The model under review builds one solid part; all positions refer to its coordinate system, in mm. A direction names the side the tool comes from. Coordinates: 2 decimals unless noted, no trailing zeros. Loops run counter-clockwise (first coordinate to the right, second up) from the corner with the lowest first, then second, coordinate; pieces in that order, holes last. Notation, with made-up numbers: M -27.75,-37 L -3.75,-37 A13 cw -3.75,-21 Z; hole C 47,6.5 d4. An arc over 180 degrees is marked long. Use one line per item in the form item = value.
```python
from build123d import *

# Parameters (mm, degrees)
SKETCH1_W                                            = 59.1
SKETCH1_H                                            = 59.1
BOSS_EXTRUDE1_DEPTH                                  = 59.1
CUT_EXTRUDE1_START                                   = -2.25
SKETCH2_W                                            = 116.357411776
SKETCH2_H                                            = 94.431830133
CUT_EXTRUDE1_DEPTH                                   = 71.232302632
FILLET1_R                                            = 7.5
SHELL1_T                                             = -2.5
CUT_EXTRUDE7_DEPTH                                   = 35
CUT_EXTRUDE8_DEPTH                                   = 35
SKETCH16_W                                           = 0.690169944
SKETCH16_H                                           = 5
CUT_EXTRUDE9_DEPTH                                   = 88.003290168
BOSS_EXTRUDE2_START                                  = 3
SKETCH18_R                                           = 5
BOSS_EXTRUDE2_DEPTH                                  = 3
SKETCH17_R                                           = 1.5
CUT_EXTRUDE10_DEPTH                                  = 10
CUT_EXTRUDE11_REACH                                  = 90.65
CSK_SLOT_FOR_M2_COUNTERSUNK_FLAT_HEAD_SC_D           = 2.4
CSK_SLOT_FOR_M2_COUNTERSUNK_FLAT_HEAD_SC_CSINK_D     = 4.4
CSK_SLOT_FOR_M2_COUNTERSUNK_FLAT_HEAD_SC_CSINK_ANGLE = 90
CSK_SLOT_FOR_M2_COUNTERSUNK_FLAT_HEA_2_D             = 2.4
CSK_SLOT_FOR_M2_COUNTERSUNK_FLAT_HEA_2_CSINK_D       = 4.4
CSK_SLOT_FOR_M2_COUNTERSUNK_FLAT_HEA_2_CSINK_ANGLE   = 90
CSK_SLOT_FOR_M2_COUNTERSUNK_FLAT_HEA_3_D             = 2.4
CSK_SLOT_FOR_M2_COUNTERSUNK_FLAT_HEA_3_CSINK_D       = 4.4
CSK_SLOT_FOR_M2_COUNTERSUNK_FLAT_HEA_3_CSINK_ANGLE   = 90
BOSS_EXTRUDE3_DEPTH                                  = 35
SKETCH28_W                                           = 7.5
SKETCH28_H                                           = 5.1
CUT_EXTRUDE12_DEPTH                                  = 62.984090748


with BuildPart() as part:
    # Sketch1 → Boss-Extrude1 (new body)
    with BuildSketch(Plane.XY):
        Rectangle(SKETCH1_W, SKETCH1_H)
    extrude(amount=BOSS_EXTRUDE1_DEPTH)

    # Sketch2 → Cut-Extrude1 (cut, through all)
    with BuildSketch(Plane(origin=(-13.400446417, -13.400446417, 19.55), x_dir=(0.9659258262890684, -0.2588190451025203, 0), z_dir=(0, 0, 1)).offset(CUT_EXTRUDE1_START)):
        with Locations((15.241895832, 15.980077556)):
            Rectangle(SKETCH2_W, SKETCH2_H)
    extrude(amount=-CUT_EXTRUDE1_DEPTH, mode=Mode.SUBTRACT)

    # Fillet1
    fillet1_edges = [part.edges().sort_by_distance(p)[0] for p in [
        (29.55, 0, 59.1),
        (0, 29.55, 59.1),
        (-29.55, 0, 59.1),
        (0, -29.55, 59.1),
        (-29.55, 29.55, 38.2),
        (29.55, 29.55, 38.2),
        (29.55, -29.55, 38.2),
        (-29.55, -29.55, 38.2),
    ]]
    fillet(fillet1_edges, radius=FILLET1_R)

    # Shell1
    shell1_openings = [part.faces().sort_by_distance(p)[0] for p in [
        (0, 0, 17.3),
    ]]
    offset(amount=SHELL1_T, openings=shell1_openings, kind=Kind.INTERSECTION)

    # Sketch14 → Cut-Extrude7 (cut)
    with BuildSketch(Plane.XY.offset(59.1)):
        Polygon((-29.55, -8.7), (-27.05, -8.7), (-27.05, -7.5), (-24.55, -7.5), (-24.55, -12.5), (-27.05, -12.5), (-27.05, -11.3), (-29.55, -11.3), align=None)
        Polygon((-29.55, 11.3), (-29.55, 8.7), (-27.05, 8.7), (-27.05, 7.5), (-24.55, 7.5), (-24.55, 12.5), (-27.05, 12.5), (-27.05, 11.3), align=None)
    extrude(amount=-CUT_EXTRUDE7_DEPTH, mode=Mode.SUBTRACT)

    # Sketch15 → Cut-Extrude8 (cut)
    with BuildSketch(Plane(origin=(-29.55, 0, -29.55), x_dir=(0, 0, -1), z_dir=(1, 0, 0))):
        Polygon((-88.65, -8.7), (-86.05, -8.7), (-86.05, -7.5), (-83.45, -7.5), (-83.45, -12.5), (-86.05, -12.5), (-86.05, -11.3), (-88.65, -11.3), align=None)
        Polygon((-88.65, 11.3), (-88.65, 8.7), (-86.05, 8.7), (-86.05, 7.5), (-83.45, 7.5), (-83.45, 12.5), (-86.05, 12.5), (-86.05, 11.3), align=None)
    extrude(amount=CUT_EXTRUDE8_DEPTH, mode=Mode.SUBTRACT)

    # Sketch16 → Cut-Extrude9 (cut, through all)
    with BuildSketch(Plane(origin=(-27.05, 0, 0), x_dir=(0, 0, -1), z_dir=(1, 0, 0))):
        with Locations((-56.845084972, -10)):
            Rectangle(SKETCH16_W, SKETCH16_H)
        with Locations((-56.845084972, 10)):
            Rectangle(SKETCH16_W, SKETCH16_H)
    extrude(amount=-CUT_EXTRUDE9_DEPTH, mode=Mode.SUBTRACT)

    # Sketch18 → Boss-Extrude2 (add)
    with BuildSketch(Plane(origin=(0, -27.05, 0), x_dir=(1, 0, 0), z_dir=(0, 1, 0)).offset(BOSS_EXTRUDE2_START)):
        with Locations((-22.05, -51.6)):
            Circle(SKETCH18_R)
    extrude(amount=-BOSS_EXTRUDE2_DEPTH)

    # Sketch17 → Cut-Extrude10 (cut)
    with BuildSketch(Plane.XZ.offset(29.55)):
        with Locations(Location((-22.05, 51.6, 0), (0, 0, 90))):
            Circle(SKETCH17_R)
    extrude(amount=-CUT_EXTRUDE10_DEPTH, mode=Mode.SUBTRACT)

    # Sketch20 → Cut-Extrude11 (cut, up to next)
    with BuildSketch(Plane.XZ.offset(29.55), mode=Mode.PRIVATE) as cut_extrude11_sk1:
        with BuildLine():
            Line((-22.647878988, 52.975696447), (-23.072143057, 53.399960516))
            Line((-23.072143057, 53.399960516), (-23.849960516, 52.622143057))
            Line((-23.849960516, 52.622143057), (-23.425696447, 52.197878988))
            ThreePointArc((-23.425696447, 52.197878988), (-23.110660172, 52.660660172), (-22.647878988, 52.975696447))
        make_face()
    cut_extrude11_tool1 = extrude(cut_extrude11_sk1.sketch, amount=-CUT_EXTRUDE11_REACH, mode=Mode.PRIVATE) & part.part
    # Sketch20 → Cut-Extrude11 (cut, up to next)
    with BuildSketch(Plane.XZ.offset(29.55), mode=Mode.PRIVATE) as cut_extrude11_sk2:
        with BuildLine():
            Line((-21.027856943, 49.800039484), (-21.452121012, 50.224303553))
            ThreePointArc((-21.452121012, 50.224303553), (-20.989339828, 50.539339828), (-20.674303553, 51.002121012))
            Line((-20.674303553, 51.002121012), (-20.250039484, 50.577856943))
            Line((-20.250039484, 50.577856943), (-21.027856943, 49.800039484))
        make_face()
    cut_extrude11_tool2 = extrude(cut_extrude11_sk2.sketch, amount=-CUT_EXTRUDE11_REACH, mode=Mode.PRIVATE) & part.part
    add(cut_extrude11_tool1.solids().sort_by_distance((-23.27308, -29.55, 52.82308))[0], mode=Mode.SUBTRACT)
    add(cut_extrude11_tool2.solids().sort_by_distance((-20.82692, -29.55, 50.37692))[0], mode=Mode.SUBTRACT)

    # CSK SLOT for M2 Countersunk Flat Head Sc (through all)
    with Locations(Plane.ZX.offset(29.55)):
        with Locations((29.55, 0)):
            CounterSinkHole(CSK_SLOT_FOR_M2_COUNTERSUNK_FLAT_HEAD_SC_D / 2, CSK_SLOT_FOR_M2_COUNTERSUNK_FLAT_HEAD_SC_CSINK_D / 2, counter_sink_angle=CSK_SLOT_FOR_M2_COUNTERSUNK_FLAT_HEAD_SC_CSINK_ANGLE)

    # CSK SLOT for M2 Countersunk Flat Hea 2 (through all)
    with Locations(Plane.XY.offset(59.1)):
        with Locations((0, 0)):
            CounterSinkHole(CSK_SLOT_FOR_M2_COUNTERSUNK_FLAT_HEA_2_D / 2, CSK_SLOT_FOR_M2_COUNTERSUNK_FLAT_HEA_2_CSINK_D / 2, counter_sink_angle=CSK_SLOT_FOR_M2_COUNTERSUNK_FLAT_HEA_2_CSINK_ANGLE)

    # CSK SLOT for M2 Countersunk Flat Hea 3 (through all)
    with Locations(Plane(origin=(0, -29.55, 0), x_dir=(-1, 0, 0), z_dir=(0, -1, 0))):
        with Locations((0, -29.55)):
            CounterSinkHole(CSK_SLOT_FOR_M2_COUNTERSUNK_FLAT_HEA_3_D / 2, CSK_SLOT_FOR_M2_COUNTERSUNK_FLAT_HEA_3_CSINK_D / 2, counter_sink_angle=CSK_SLOT_FOR_M2_COUNTERSUNK_FLAT_HEA_3_CSINK_ANGLE)

    # Sketch27 → Boss-Extrude3 (add)
    with BuildSketch(Plane(origin=(-29.55, 29.55, 0), x_dir=(0, 0, -1), z_dir=(1, 0, 0))):
        Polygon((-18.3, -59.1), (-18.3, -61.7), (-17.05, -61.7), (-17.05, -64.2), (-22.05, -64.2), (-22.05, -61.7), (-20.8, -61.7), (-20.8, -59.1), align=None)
        Polygon((-38.3, -59.1), (-40.8, -59.1), (-40.8, -61.7), (-42.05, -61.7), (-42.05, -64.2), (-37.05, -64.2), (-37.05, -61.7), (-38.3, -61.7), align=None)
    extrude(amount=BOSS_EXTRUDE3_DEPTH)

    # Sketch28 → Cut-Extrude12 (cut, through all)
    with BuildSketch(Plane.XY.offset(59.1)):
        with Locations((-25.8, -32.1)):
            Rectangle(SKETCH28_W, SKETCH28_H)
    extrude(amount=-CUT_EXTRUDE12_DEPTH, mode=Mode.SUBTRACT)


solid = part.part
```
1. Machinability: for faces 1 (the face through (-10, -8.7, 58)), 2 (the face through (-8, -33, 37.05)), 3 (the face through (-18.42, -25.53, 48.16)), 4 (the face through (-23, -24.05, 50)), which of the approach directions +Z, -Z, +X, -X, +Y, -Y give a long, thin tool a straight path to every point of the face, cutting with its end or side? Answer none if there is none.
Response values:
face_1 = +Z, -Z, -X
face_2 = +X, -X, -Y
face_3 = none
face_4 = -Z
2. Add section C-C (z = 29.55). Count the separate pieces of the cut face and the enclosed holes in it, then the cut area to 3 significant figures.
Response values:
separate_pieces = 4
enclosed_holes = 0
area = 512 mm^2
3. The part is to be moulded in two halves that separate along Z. For faces 5 (the face through (-22.05, -33, 40)), 6 (the face through (-8, -31, 40.8)), 7 (the face through (-8, -31, 38.3)), say which applies: pulls with the +Z half, pulls with the -Z half, needs draft (parallel to the pull), parting line crosses it, or undercut.
Response values:
face_5 = needs draft
face_6 = pulls with the +Z half
face_7 = undercut
4. Insertion check: P1, Ø1.5, axis at y = -32.5, z = 19.5, coming from the +X side; P2, Ø2, axis at x = -18.5, y = 2.5, coming from the -Z side; P3, Ø1.3, axis at x = -28.5, z = 46, coming from the +Y side (3 decimals). Each pin has a flat end and moves straight along its axis. Give the tip position at first contact, or say it passes through.
Response values:
P1 = 5.45
P2 = 56.6
P3 = 26.805
5. Wall thickness on line 1 along Y through (x, z) = (11.5, 40); line 2 along Y through (x, z) = (-8.5, 42): over which ranges is each line inside the solid? List them lowest first. Write a range as from..to.
Response values:
line_1 = -29.55..-27.05, 27.05..29.55
line_2 = -34.65..-32.15, -29.55..-27.05, 27.05..29.55
6. Add section A-A (y = 0). State the section outline as (x, z) points, then the cut area to 3 significant figures.
Response values:
outline = M -29.55,17.3 L -27.05,17.3 L -27.05,51.6 A5 cw -22.05,56.6 L -1.2,56.6 L -1.2,58.1 L -2.2,59.1 L -22.05,59.1 A7.5 ccw -29.55,51.6 Z; M 1.2,56.6 L 22.05,56.6 A5 cw 27.05,51.6 L 27.05,17.3 L 29.55,17.3 L 29.55,51.6 A7.5 ccw 22.05,59.1 L 2.2,59.1 L 1.2,58.1 Z
area = 324 mm^2
7. Add section B-B (x = 18.5). State the section outline as (y, z) points, then the cut area to 3 significant figures.
Response values:
outline = M -29.55,17.3 L -27.05,17.3 L -27.05,51.6 A5 cw -22.05,56.6 L 22.05,56.6 A5 cw 27.05,51.6 L 27.05,17.3 L 29.55,17.3 L 29.55,51.6 A7.5 ccw 22.05,59.1 L -22.05,59.1 A7.5 ccw -29.55,51.6 Z
area = 331 mm^2
